```python
from build123d import *

# Parameters (mm, degrees)
SKETCH2_W           = 53.975
SKETCH2_H           = 31.75
SKETCH2_R           = 1
SKETCH2_W_2         = 5.08
SKETCH2_H_2         = 16.51
BOSS_EXTRUDE1_DEPTH = 3.175
SKETCH3_R           = 6.35
CUT_EXTRUDE1_DEPTH  = 3.175
SKETCH4_R           = 1.778
CUT_EXTRUDE2_DEPTH  = 3.175
CIRPATTERN1_COUNT   = 4
FILLET1_R           = 2.54


with BuildPart() as part:
    # Sketch2 → Boss-Extrude1 (new body)
    with BuildSketch(Plane.XY):
        with Locations((26.9875, 15.875)):
            Rectangle(SKETCH2_W, SKETCH2_H)
        with Locations((32.385, 26.67)):
            Circle(SKETCH2_R, mode=Mode.SUBTRACT)
        with Locations((47.625, 26.67)):
            Circle(SKETCH2_R, mode=Mode.SUBTRACT)
        with Locations((32.385, 5.08)):
            Circle(SKETCH2_R, mode=Mode.SUBTRACT)
        with Locations((47.625, 5.08)):
            Circle(SKETCH2_R, mode=Mode.SUBTRACT)
        with Locations((31.75, 15.875)):
            Rectangle(SKETCH2_W_2, SKETCH2_H_2, mode=Mode.SUBTRACT)
        with Locations((48.133, 15.875)):
            Rectangle(SKETCH2_W_2, SKETCH2_H_2, mode=Mode.SUBTRACT)
    extrude(amount=BOSS_EXTRUDE1_DEPTH)

    # Sketch3 → Cut-Extrude1 (cut)
    with BuildSketch(Plane.XY.offset(3.175)):
        with Locations((12.7, 15.875)):
            Circle(SKETCH3_R)
    extrude(amount=-CUT_EXTRUDE1_DEPTH, mode=Mode.SUBTRACT)

    # Sketch4 → Cut-Extrude2 (cut)
    with BuildSketch(Plane.XY.offset(3.175)):
        with Locations((12.7, 25.654)):
            Circle(SKETCH4_R)
    cut_extrude2 = extrude(amount=-CUT_EXTRUDE2_DEPTH, mode=Mode.SUBTRACT)

    # CirPattern1: Cut-Extrude2 ×4 about axis
    cirpattern1_axis = Axis((12.7, 15.875, 0), (0, 0, 1))
    for i in range(1, CIRPATTERN1_COUNT):
        add(cut_extrude2.rotate(cirpattern1_axis, i * 360 / CIRPATTERN1_COUNT), mode=Mode.SUBTRACT)

    # Fillet1
    fillet1_edges = [part.edges().sort_by_distance(p)[0] for p in [
        (0, 31.75, 1.5875),
        (53.975, 31.75, 1.5875),
        (53.975, 0, 1.5875),
        (0, 0, 1.5875),
    ]]
    fillet(fillet1_edges, radius=FILLET1_R)


solid = part.part
```
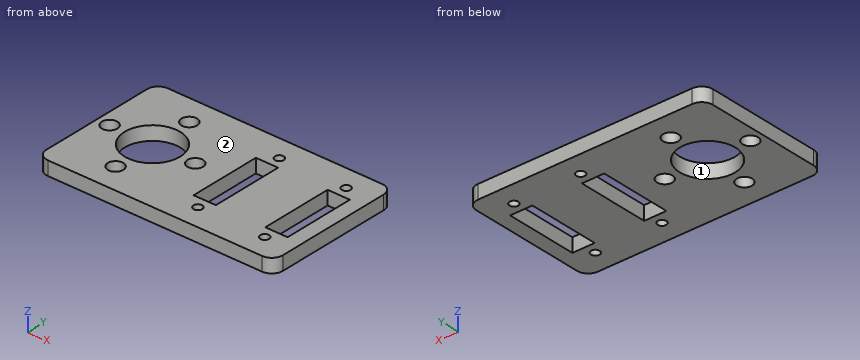
Can you work these out from the model? Positions are in its coordinate system, mm. Face numbers are marked on the shaded views. Round coordinates to 2 decimals unless told otherwise and drop trailing zeros. Order: outer loops, then holes, each group sorted by start corner. A loop starts at its lowest first (then second) coordinate and runs counter-clockwise, first axis right, second up.
(1) If I drill on L1, parallel to X at y = 23.5, z = 0.3 (3 decimals); L2, parallel to Y at x = 12.7, z = 2.25 (3 decimals); L3, parallel to X at y = 26.5, z = 1.65 (3 decimals), over which ranges is the centre line in solid material (lowest first)?
Results are:
L1: x = 0 to 29.21, 34.29 to 45.593, 50.673 to 53.975
L2: y = 0 to 4.318, 7.874 to 9.525, 22.225 to 23.876, 27.432 to 31.75
L3: x = 0 to 11.136, 14.264 to 31.4, 33.37 to 46.64, 48.61 to 53.975
(2) If we section it at C-C (z = 0.8): Count the separate pieces of the cut face and the enclosed holes in it, plus the area to 3 significant figures.
Results are:
separate pieces: 1
enclosed holes: 11
area: 1,360 mm2
(3) If we section it at D-D (y = 26.67): Please give me the cut outline in (x, z) (3 decimals).
Results are:
outline: (0, 0) - (11.241, 0) - (11.241, 3.175) - (0, 3.175) - close; (14.159, 0) - (31.385, 0) - (31.385, 3.175) - (14.159, 3.175) - close; (33.385, 0) - (46.625, 0) - (46.625, 3.175) - (33.385, 3.175) - close; (48.625, 0) - (53.975, 0) - (53.975, 3.175) - (48.625, 3.175) - close
(4) If we section it at A-A (y = 12.5): Please give me the cut outline in (x, z) (3 decimals).
Results are:
outline: (0, 0) - (7.321, 0) - (7.321, 3.175) - (0, 3.175) - close; (18.079, 0) - (29.21, 0) - (29.21, 3.175) - (18.079, 3.175) - close; (34.29, 0) - (45.593, 0) - (45.593, 3.175) - (34.29, 3.175) - close; (50.673, 0) - (53.975, 0) - (53.975, 3.175) - (50.673, 3.175) - close
(5) We'd pull the mould along Y, two halves only. Please class the marked faces 1 and 2: +Y half, -Y half, draft (parallel to the pull), parting line (faces both ways), or undercut.
Results are:
face 1: undercut
face 2: draft
(6) I'm going to push a flat-ended pin straight in: pin 1 (2 mm diameter, centred on x = 2.921, y = 15.875, fed in from -Z). Where does the tip first touch, or does it pass through?
Results are:
pin 1: passes through
(7) If we section it at B-B (x = 4): Please give me the cut outline in (y, z) (3 decimals), plus the area to 3 significant figures.
Results are:
outline: (0, 0) - (14.462, 0) - (14.462, 3.175) - (0, 3.175) - close; (17.288, 0) - (31.75, 0) - (31.75, 3.175) - (17.288, 3.175) - close
area: 91.8 mm2
